Source: CAD feature listing. Evaluate the final solid. Frame: model axes, mm. Face numbers are marked on the shaded views. A direction names the side the tool comes from. Give positions to 0.01 mm unless a question says otherwise; leave off trailing zeros. Order: outer loops, then holes, each group sorted by start corner. A loop starts at its lowest first (then second) coordinate and runs counter-clockwise, first axis right, second up.
1) Material intervals for line 1 (Z direction, x = 31, y = 18.5); line 2 (X direction, y = 21, z = 16.5); line 3 (Z direction, x = 4, y = 27), sorted ascending.
2) Section D-D, the plane z = 35. Return loops of the section in (x, y).
3) First-contact query: P1, Ø11, axis at y = 18.5, z = 26.5, coming from the -X side; P2, Ø7.5, axis at x = 12.5, y = 5.5, coming from the +Z side; P3, Ø1.5, axis at y = 22, z = 31, coming from the +X side. Flat tips, straight axial feed; report the tip coordinate or a pass-through.
4) Section B-B, the plane x = 22. Return loops of the section in (y, z), plus the area to 3 significant figures.
5) Draft query along Y for the marked faces 4, 5, 6 and 7. Return one class per face: released by +Y, released by -Y, zero draft, split by the parting line, or undercut.
6) Section C-C, the plane y = 27. Return loops of the section in (x, z).
7) Access query for the marked faces 1, 2 and 3. Directions: +Z, -Z, +X, -X, +Y, -Y. A direction counts if a zero-diameter tool reaches every point of the face in a straight line with its end or side. Return the directions, or none.
8) Section A-A, the plane z = 23. Return loops of the section in (x, y), plus the area to 3 significant figures.
```python
from build123d import *

# Parameters (mm, degrees)
SKETCH1_W            = 40
SKETCH1_H            = 40
BOSS_EXTRUDE1_DEPTH  = 40
SKETCH2_W            = 10
SKETCH2_H            = 10
CUT_EXTRUDE1_DEPTH   = 40
SKETCH4_W            = 10
SKETCH4_H            = 10
SKETCH4_H_2          = 30
CUT_EXTRUDE2_DEPTH   = 40
SKETCH5_W            = 20
SKETCH5_H            = 10
CUT_EXTRUDE3_DEPTH   = 10
SKETCH7_W            = 20
SKETCH7_H            = 10
CUT_EXTRUDE16_DEPTH  = 20
SKETCH11_W           = 20
SKETCH11_H           = 20
CUT_EXTRUDE19_DEPTH  = 10
CUT_EXTRUDE20_DEPTH  = 10
SKETCH13_W           = 20
SKETCH13_H           = 10
CUT_EXTRUDE21_DEPTH  = 10
BOSS_EXTRUDE2_DEPTH  = 10
SKETCH16_W           = 20
SKETCH16_H           = 20
CUT_EXTRUDE25_DEPTH  = 10
CUT_EXTRUDE26_DEPTH  = 10
SKETCH22_W           = 20
SKETCH22_H           = 10
BOSS_EXTRUDE5_DEPTH  = 10
BOSS_EXTRUDE6_DEPTH  = 10
SKETCH24_W           = 20
SKETCH24_H           = 20
BOSS_EXTRUDE7_DEPTH  = 10
BOSS_EXTRUDE8_DEPTH  = 10
BOSS_EXTRUDE9_DEPTH  = 10
CUT_EXTRUDE27_DEPTH  = 10
BOSS_EXTRUDE12_DEPTH = 10
CUT_EXTRUDE30_DEPTH  = 20
CUT_EXTRUDE31_DEPTH  = 10
SKETCH32_W           = 10
SKETCH32_H           = 19.95
CUT_EXTRUDE36_DEPTH  = 10
SKETCH33_W           = 0.033333333
SKETCH33_H           = 10
CUT_EXTRUDE37_DEPTH  = 10
BOSS_EXTRUDE13_DEPTH = 10
CUT_EXTRUDE40_DEPTH  = 20


with BuildPart() as part:
    # Sketch1 → Boss-Extrude1 (new body)
    with BuildSketch(Plane.XY):
        with Locations((20, 20)):
            Rectangle(SKETCH1_W, SKETCH1_H)
    extrude(amount=BOSS_EXTRUDE1_DEPTH)

    # Sketch2 → Cut-Extrude1 (cut)
    with BuildSketch(Plane.XY.offset(40)):
        with Locations((5, 35)):
            Rectangle(SKETCH2_W, SKETCH2_H)
    extrude(amount=-CUT_EXTRUDE1_DEPTH, mode=Mode.SUBTRACT)

    # Sketch4 → Cut-Extrude2 (cut)
    with BuildSketch(Plane(origin=(0, 40, 0), x_dir=(1, 0, 0), z_dir=(0, 1, 0))):
        with Locations((35, -35)):
            Rectangle(SKETCH4_W, SKETCH4_H)
        with Locations((5, -25)):
            Rectangle(SKETCH4_W, SKETCH4_H_2)
    extrude(amount=-CUT_EXTRUDE2_DEPTH, mode=Mode.SUBTRACT)

    # Sketch5 → Cut-Extrude3 (cut)
    with BuildSketch(Plane.XY.offset(40)):
        with Locations((20, 5)):
            Rectangle(SKETCH5_W, SKETCH5_H)
    extrude(amount=-CUT_EXTRUDE3_DEPTH, mode=Mode.SUBTRACT)

    # Sketch7 → Cut-Extrude16 (cut)
    with BuildSketch(Plane.XY.offset(40)):
        with Locations((20, 35)):
            Rectangle(SKETCH7_W, SKETCH7_H)
    extrude(amount=-CUT_EXTRUDE16_DEPTH, mode=Mode.SUBTRACT)

    # Sketch11 → Cut-Extrude19 (cut)
    with BuildSketch(Plane.XY.offset(40)):
        with Locations((20, 20)):
            Rectangle(SKETCH11_W, SKETCH11_H)
    extrude(amount=-CUT_EXTRUDE19_DEPTH, mode=Mode.SUBTRACT)

    # Sketch12 → Cut-Extrude20 (cut)
    with BuildSketch(Plane(origin=(0, 0, 0), x_dir=(-1, 0, 0), z_dir=(0, 0, -1))):
        Polygon((-10, 30), (-40, 40), (-10, 40), align=None)
    extrude(amount=-CUT_EXTRUDE20_DEPTH, mode=Mode.SUBTRACT)

    # Sketch13 → Cut-Extrude21 (cut)
    with BuildSketch(Plane.XY.offset(20)):
        with Locations((20, 35)):
            Rectangle(SKETCH13_W, SKETCH13_H)
    extrude(amount=-CUT_EXTRUDE21_DEPTH, mode=Mode.SUBTRACT)

    # Sketch15 → Boss-Extrude2 (add)
    with BuildSketch(Plane(origin=(0, 0, 0), x_dir=(-1, 0, 0), z_dir=(0, 0, -1))):
        Polygon((-40, 40), (-10, 40), (-10, 30), align=None)
    extrude(amount=-BOSS_EXTRUDE2_DEPTH)

    # Sketch16 → Cut-Extrude25 (cut)
    with BuildSketch(Plane.XY.offset(30)):
        with Locations((20, 20)):
            Rectangle(SKETCH16_W, SKETCH16_H)
    extrude(amount=-CUT_EXTRUDE25_DEPTH, mode=Mode.SUBTRACT)

    # Sketch19 → Cut-Extrude26 (cut)
    with BuildSketch(Plane.XY.offset(30)):
        Polygon((10, 0), (30, 30), (10, 30), align=None)
    extrude(amount=-CUT_EXTRUDE26_DEPTH, mode=Mode.SUBTRACT)

    # Sketch22 → Boss-Extrude5 (add)
    with BuildSketch(Plane.XY.offset(10)):
        with Locations((20, 35)):
            Rectangle(SKETCH22_W, SKETCH22_H)
    extrude(amount=BOSS_EXTRUDE5_DEPTH)

    # Sketch23 → Boss-Extrude6 (add)
    with BuildSketch(Plane.XY.offset(20)):
        Polygon((16.666666667, 10), (10, 10), (10, 0), align=None)
    extrude(amount=BOSS_EXTRUDE6_DEPTH)

    # Sketch24 → Boss-Extrude7 (add)
    with BuildSketch(Plane.XY.offset(20)):
        with Locations((20, 20)):
            Rectangle(SKETCH24_W, SKETCH24_H)
    extrude(amount=BOSS_EXTRUDE7_DEPTH)

    # Sketch25 → Boss-Extrude8 (add)
    with BuildSketch(Plane.XY.offset(30)):
        Polygon((10, 0), (30, 30), (10, 30), align=None)
    extrude(amount=BOSS_EXTRUDE8_DEPTH)

    # Sketch26 → Boss-Extrude9 (add)
    with BuildSketch(Plane.XY.offset(30)):
        Polygon((30, 30), (30, 10), (16.666666667, 10), align=None)
    extrude(amount=BOSS_EXTRUDE9_DEPTH)

    # Sketch27 → Cut-Extrude27 (cut)
    with BuildSketch(Plane.XY.offset(40)):
        Polygon((10, 0), (30, 30), (10, 30), align=None)
    extrude(amount=-CUT_EXTRUDE27_DEPTH, mode=Mode.SUBTRACT)

    # Sketch28 → Boss-Extrude12 (add)
    with BuildSketch(Plane.XY.offset(30)):
        Polygon((10, 10), (16.666666667, 10), (30, 30), (10, 30), align=None)
        Polygon((10, 0), (16.666666667, 10), (10, 10), align=None)
    extrude(amount=BOSS_EXTRUDE12_DEPTH)

    # Sketch29 → Cut-Extrude30 (cut)
    with BuildSketch(Plane.XY.offset(40)):
        Polygon((29.966666667, 29.95), (16.666666667, 10), (29.966666667, 10), align=None)
    extrude(amount=-CUT_EXTRUDE30_DEPTH, mode=Mode.SUBTRACT)

    # Sketch30 → Cut-Extrude31 (cut)
    with BuildSketch(Plane.XY.offset(40)):
        Polygon((30, 30), (10, 30), (10, 10), (16.666666667, 10), align=None)
    extrude(amount=-CUT_EXTRUDE31_DEPTH, mode=Mode.SUBTRACT)

    # Sketch32 → Cut-Extrude36 (cut)
    with BuildSketch(Plane.ZY.offset(-29.966666667)):
        with Locations((35, 19.975)):
            Rectangle(SKETCH32_W, SKETCH32_H)
    extrude(amount=-CUT_EXTRUDE36_DEPTH, mode=Mode.SUBTRACT)

    # Sketch33 → Cut-Extrude37 (cut)
    with BuildSketch(Plane.XZ.offset(-29.95)):
        with Locations((29.983333334, 35)):
            Rectangle(SKETCH33_W, SKETCH33_H)
    extrude(amount=-CUT_EXTRUDE37_DEPTH, mode=Mode.SUBTRACT)

    # Sketch34 → Boss-Extrude13 (add)
    with BuildSketch(Plane.XY.offset(30)):
        Polygon((10, 10), (16.666666667, 10), (30, 30), (10, 30), align=None)
    extrude(amount=BOSS_EXTRUDE13_DEPTH)

    # Sketch35 → Cut-Extrude40 (cut)
    with BuildSketch(Plane.XY.offset(40)):
        Polygon((10, 0), (10, 9.999), (16.666, 9.999), align=None)
    extrude(amount=-CUT_EXTRUDE40_DEPTH, mode=Mode.SUBTRACT)


solid = part.part
```
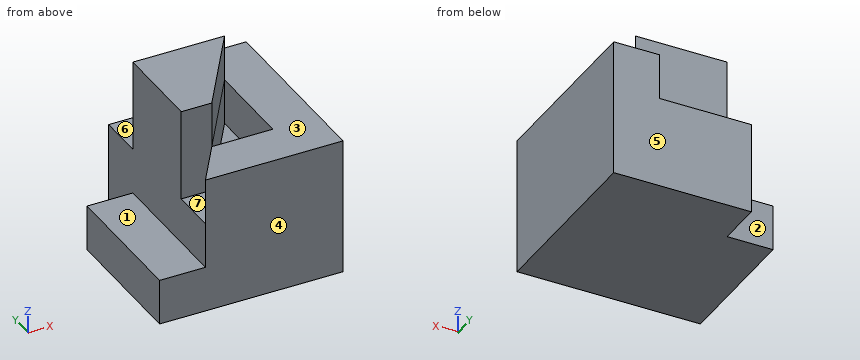
From the geometry:
1. line 1: z = 0 to 30
1. line 2: x = 10 to 40
1. line 3: z = 0 to 10
2. outline: (10, 10) - (16.67, 10) - (30, 30) - (10, 30) - close
3. P1: stops at x = 10
3. P2: stops at z = 30
3. P3: stops at x = 25.17
4. outline: (0, 0) - (40, 0) - (40, 20) - (30, 20) - (30, 40) - (18, 40) - (18, 20) - (10, 20) - (10, 30) - (0, 30) - close
4. area: 1,140 mm2
5. face 4: released by -Y
5. face 5: released by +Y
5. face 6: zero draft
5. face 7: undercut
6. outline: (0, 0) - (40, 0) - (40, 30) - (29.97, 30) - (29.97, 20) - (28, 20) - (28, 40) - (10, 40) - (10, 10) - (0, 10) - close
7. face 1: +Z, -X, +Y, -Y
7. face 2: +Z, -Z, -X, +Y
7. face 3: +Z, +X, -Y
8. outline: (10, 0) - (40, 0) - (40, 40) - (30, 40) - (30, 30) - (10, 30) - (10, 10) - (16.67, 10) - close; hole (16.67, 10) - (29.97, 10) - (29.97, 29.95) - close
8. area: 834 mm2
